Geometry: final body of the model. Coordinates: model frame, mm. A direction names the side the tool comes from. Coordinates: 2 decimals unless noted, no trailing zeros. Write each loop counter-clockwise with the first axis right and the second up, starting at its lowest first coordinate (ties: lowest second). Pieces come first, ordered by that corner, then holes. Notation, with made-up numbers: (33, 26) -> (67, 26) arc R20 ccw to (67, 57) -> close; hole circle Ø5 at (-19, 86.25). An arc over 180 degrees is marked (long way). One line per item, written item: value.
```python
from build123d import *

# Parameters (mm, degrees)
SKETCH1_R           = 3
BOSS_EXTRUDE1_DEPTH = 10
FILLET2_R           = 60
FILLET3_R           = 70


with BuildPart() as part:
    # Sketch1 → Boss-Extrude1 (new body)
    with BuildSketch(Plane(origin=(0, 0, 0), x_dir=(1, 0, 0), z_dir=(0, 1, 0))):
        Polygon((165, -120), (85, -120), (85, -15), (102, -15), (102, 125), (255, 125), (255, 15), (165, 15), align=None)
        with Locations(Location((146.4, -101.4, 0), (0, 0, 270))):
            Circle(SKETCH1_R, mode=Mode.SUBTRACT)
        with Locations(Location((106.4, -101.4, 0), (0, 0, 270))):
            Circle(SKETCH1_R, mode=Mode.SUBTRACT)
        with Locations(Location((146.4, -61.4, 0), (0, 0, 270))):
            Circle(SKETCH1_R, mode=Mode.SUBTRACT)
        with Locations(Location((106.4, -61.4, 0), (0, 0, 270))):
            Circle(SKETCH1_R, mode=Mode.SUBTRACT)
        with Locations(Location((122, 35, 0), (0, 0, 270))):
            Circle(SKETCH1_R, mode=Mode.SUBTRACT)
        with Locations(Location((235, 35, 0), (0, 0, 270))):
            Circle(SKETCH1_R, mode=Mode.SUBTRACT)
        with Locations(Location((235, 105, 0), (0, 0, 270))):
            Circle(SKETCH1_R, mode=Mode.SUBTRACT)
        with Locations(Location((122, 105, 0), (0, 0, 270))):
            Circle(SKETCH1_R, mode=Mode.SUBTRACT)
    extrude(amount=BOSS_EXTRUDE1_DEPTH)

    # Fillet2
    # the kernel refuses this fillet: 60 mm, written as the material it adds along each edge
    with BuildSketch(Plane(origin=(102, 0, 15), x_dir=(-1, 0, 0), z_dir=(0, 1, 0))) as fillet2_piece_1:
        with BuildLine():
            CenterArc((60, -41.844951906), FILLET2_R, 135.779955572, 44.220044428)
            Line((0, -41.844951906), (-1.2, -41.844951906))
            Line((-1.2, -41.844951906), (-1.2, 0))
            Line((-1.2, 0), (0, 1.2))
            ThreePointArc((0, 1.2), (8.5, 1.2), (16.14, 0.836899038))
            Line((16.14, 0.836899038), (17, 0))
        make_face()
    extrude(amount=10)

    # Fillet3
    fillet3_edges = [part.edges().sort_by_distance(p)[0] for p in [
        (85, 5, 15),
    ]]
    fillet(fillet3_edges, radius=FILLET3_R)


solid = part.part
```
(1) Section D-D (x = 223.5). Return the cut outline in (y, z).
Responses:
outline: (0, -125) -> (10, -125) -> (10, -15) -> (0, -15) -> close
(2) Section C-C (y = 5). State how many separate pieces and enclosed holes the cut face has, then the cut area to 3 significant figures.
Responses:
separate pieces: 1
enclosed holes: 8
area: 27,100 mm2
(3) Reachability of faces 1 (the flat face through (150, 10, -28)), 2 (the flat face through (102, 5, -75)), 3 (the flat face through (211, 5, -15)) from +Z, -Z, +X, -X, +Y, -Y: full face, straight path, thin tool, end or side. Return the list, or none.
Responses:
face 1: +Z, -Z, +X, -X, +Y
face 2: -Z, -X, +Y, -Y
face 3: +Z, +X, +Y, -Y
(4) Pull-direction query (Z, two-part tool) for faces 4 (the cylindrical face through (124.03, 4.93, -37.21)), 5 (the cylindrical face through (87.392, 5.07, 19.284)), 6 (the cylindrical face through (124.03, 4.93, -107.21)), 7 (the flat face through (165, 5, 52)); classes: released by +Z, released by -Z, zero draft, split by the parting line, or undercut.
Responses:
face 4: undercut
face 5: released by -Z
face 6: undercut
face 7: zero draft
(5) Section A-A (x = 106.4). Return the cut outline in (y, z).
Responses:
outline: (0, -125) -> (10, -125) -> (10, 58.4) -> (0, 58.4) -> close; (0, 64.4) -> (10, 64.4) -> (10, 98.4) -> (0, 98.4) -> close; (0, 104.4) -> (10, 104.4) -> (10, 120) -> (0, 120) -> close
(6) Section B-B (z = -35). Return the cut outline in (x, y), then the cut area to 3 significant figures.
Responses:
outline: (102, 0) -> (119, 0) -> (119, 10) -> (102, 10) -> close; (125, 0) -> (232, 0) -> (232, 10) -> (125, 10) -> close; (238, 0) -> (255, 0) -> (255, 10) -> (238, 10) -> close
area: 1,410 mm2
(7) Line query: line 1 (Z direction, x = 146.4, y = 3); line 2 (Z direction, x = 235, y = 6.5); line 3 (X direction, y = 8, z = -105). Output: solid intervals per line, ascending. Write a range as [from, to].
Responses:
line 1: z = [-125, 58.4], [64.4, 98.4], [104.4, 120]
line 2: z = [-125, -108], [-102, -38], [-32, -15]
line 3: x = [102, 119], [125, 232], [238, 255]
(8) First-contact query: pin 1 (5.5 mm diameter, centred on x = 235, z = -105, fed in from -Y) (1 decimal); pin 2 (7 mm diameter, centred on x = 146.4, z = 61.4, fed in from +Y); pin 3 (2 mm diameter, centred on x = 215, y = 3, fed in from +Z). Flat tips, straight axial feed; report the tip coordinate or a pass-through.
Responses:
pin 1: passes through
pin 2: stops at y = 10
pin 3: stops at z = -15
